from build123d import *

# Parameters (mm, degrees)
CROQUIS1_R                 = 8
SALIENTE_EXTRUIR1_DEPTH    = 30
CORTAR_EXTRUIR1_DEPTH      = 8.5
CROQUIS9_R                 = 12.5
SALIENTE_EXTRUIR5_DEPTH    = 20
CROQUIS3_R                 = 10.95
CORTAR_EXTRUIR2_DEPTH      = 19
CORTAR_EXTRUIR3_REACH      = 27.952
CROQUIS4_R                 = 2.025
CORTAR_EXTRUIR4_DEPTH      = 35.820970693
CORTAR_EXTRUIR4_DEPTH_BACK = 35.820970693
CROQUIS5_R                 = 2
CROQUIS7_R                 = 8
SALIENTE_EXTRUIR3_DEPTH    = 3
REDONDEO1_R                = 10


with BuildPart() as part:
    # Croquis1 → Saliente-Extruir1 (new body)
    with BuildSketch(Plane(origin=(0, 0, 0), x_dir=(0, 0, -1), z_dir=(1, 0, 0))):
        Circle(CROQUIS1_R)
    extrude(amount=SALIENTE_EXTRUIR1_DEPTH)

    # Croquis2 → Cortar-Extruir1 (cut)
    with BuildSketch(Plane(origin=(30, 0, 0), x_dir=(0, 0, -1), z_dir=(1, 0, 0))):
        Polygon((0, -6.957070744), (6.025, -3.478535372), (6.025, 3.478535372), (0, 6.957070744), (-6.025, 3.478535372), (-6.025, -3.478535372), align=None)
    extrude(amount=-CORTAR_EXTRUIR1_DEPTH, mode=Mode.SUBTRACT)

    # Croquis9 → Saliente-Extruir5 (add)
    with BuildSketch(Plane.ZY):
        Circle(CROQUIS9_R)
    extrude(amount=-SALIENTE_EXTRUIR5_DEPTH)

    # Croquis3 → Cortar-Extruir2 (cut)
    with BuildSketch(Plane.ZY):
        Circle(CROQUIS3_R)
    extrude(amount=-CORTAR_EXTRUIR2_DEPTH, mode=Mode.SUBTRACT)

    # Croquis4 → Cortar-Extruir3 (cut, up to next)
    with BuildSketch(Plane.ZY.offset(-19), mode=Mode.PRIVATE) as cortar_extruir3_sk1:
        Circle(CROQUIS4_R)
    cortar_extruir3_tool1 = extrude(cortar_extruir3_sk1.sketch, amount=-CORTAR_EXTRUIR3_REACH, mode=Mode.PRIVATE) & part.part
    add(cortar_extruir3_tool1.solids().sort_by_distance((19, 0, 0))[0], mode=Mode.SUBTRACT)

    # Croquis5 → Cortar-Extruir4 (cut, two sides: drawn at the far end of the back side and taken through both)
    with BuildSketch(Plane.XY.offset(-CORTAR_EXTRUIR4_DEPTH_BACK)):
        with Locations((6, 0)):
            Circle(CROQUIS5_R)
    extrude(amount=CORTAR_EXTRUIR4_DEPTH + CORTAR_EXTRUIR4_DEPTH_BACK, mode=Mode.SUBTRACT)

    # Croquis7 → Saliente-Extruir3 (add)
    with BuildSketch(Plane(origin=(30, 0, 0), x_dir=(0, 0, -1), z_dir=(1, 0, 0))):
        with Locations(Location((0, 0, 0), (0, 0, 180))):
            Circle(CROQUIS7_R)
        Polygon((-6.025, -3.478535372), (0, -6.957070744), (6.025, -3.478535372), (6.025, 3.478535372), (0, 6.957070744), (-6.025, 3.478535372), align=None, mode=Mode.SUBTRACT)
    extrude(amount=SALIENTE_EXTRUIR3_DEPTH)

    # Redondeo1
    # the kernel refuses this fillet: 10 mm, written as the material it adds along each edge
    with BuildSketch(Plane(origin=(20, 0, 0), x_dir=(0, 0, -1), z_dir=(0, 1, 0))) as redondeo1_piece_1:
        with BuildLine():
            CenterArc((18, -8.351646544), REDONDEO1_R, 123.367012969, 56.632987031)
            Line((12.5, 0), (12.39, 0.167032931))
            ThreePointArc((12.39, 0.167032931), (10.25, 0.2), (8, 0.2))
            Line((8, 0.2), (7.8, 0))
            Line((7.8, 0), (7.8, -8.351646544))
            Line((7.8, -8.351646544), (8, -8.351646544))
        make_face()
    revolve(axis=Axis((20, 0, 0), (-1, 0, 0)))


solid = part.part
Read the model definition and answer for the solid it produces. Units are mm, in the model's axes. A direction names the side the tool comes from. Coordinates: 2 decimals unless noted, no trailing zeros. Order: outer loops, then holes, each group sorted by start corner. A loop starts at its lowest first (then second) coordinate and runs counter-clockwise, first axis right, second up. Notation, with made-up numbers: M -4.75,88 L 35.25,88 A25 ccw 35.25,114 Z; hole C 20.25,39 d6. An arc over 180 degrees is marked long. Put each result on its own line as item: value. Start each with the question number.
Item 1: Section A-A, the plane x = 30.5 is taken. Determine the outline of the cut face in (y, z) (3 decimals), plus the area to 3 significant figures.
Item 2: Consider probe 1 along Z at (x, y) = (13.75, 0); probe 2 along X at (y, z) = (2.75, -0.5); probe 3 along Y at (x, z) = (27, -5.5). Determine where each line is inside the solid, lowest interval first. Write a range as [from, to].
Item 3: Section C-C, the plane x = 11 is taken. Determine the outline of the cut face in (y, z).
Item 4: Given pin 1 Ø1.5 at (x, y) = (10.5, -3.5) entering from +Z; pin 2 Ø5.5 at (x, y) = (26, 0.5) entering from -Z; pin 3 Ø10 at (x, z) = (25, -6) entering from +Y; pin 4 Ø2.5 at (x, y) = (6, 0) entering from +Z, each flat-ended and moving along its own axis, determine where each tip first touches the part or whether it passes through.
Item 5: For faces 4 (the face through (33, 5, -4)), 5 (the face through (27.17, -5.193, 3.055)), 6 (the face through (19, 0.2, 2.3)), determine the directions among +Z, -Z, +X, -X, +Y, -Y from which every point of the face is accessible in a straight line to the end or side of a thin tool.
Item 6: Section D-D, the plane x = 21 is taken. Determine the outline of the cut face in (y, z) (3 decimals), plus the area to 3 significant figures.
Item 7: The mould has two halves that part along Z. Classify faces 1 (the face through (0, -11.1, -0.1)), 2 (the face through (27.17, -5.242, -2.97)), 3 (the face through (9.86, 3.755, 11.923)): +Z half, -Z half, draft (parallel to the pull), parting line (faces both ways), or undercut.
Item 8: Section B-B, the plane x = 6 is taken. Determine the outline of the cut face in (y, z).
Computed:
1. outline: C 0,0 d16; hole M -6.957,0 L -3.479,-6.025 L 3.479,-6.025 L 6.957,0 L 3.479,6.025 L -3.479,6.025 Z
1. area: 75.3 mm2
2. probe 1: z = [-12.5, -10.95], [10.95, 12.5]
2. probe 2: x = [19, 21.5]
2. probe 3: y = [-5.94, -3.78], [3.78, 5.94]
3. outline: C 0,0 d25; hole C 0,0 d21.9
4. pin 1: stops at z = 12.19
4. pin 2: stops at z = -9.39
4. pin 3: stops at y = 11.31
4. pin 4: passes through
5. face 4: +Z, -Z, +X, +Y, -Y
5. face 5: +X
5. face 6: -X
6. outline: C 0,0 d22.442; hole C 0,0 d4.05
6. area: 383 mm2
7. face 1: draft
7. face 2: undercut
7. face 3: parting line
8. outline: M -2,-12.34 L -2,-10.77 A10.95 cw -2,10.77 L -2,12.34 A12.5 ccw Z; M 2,-12.34 A12.5 ccw 2,12.34 L 2,10.77 A10.95 cw 2,-10.77 Z
